Build history of the part. All positions in model axes, mm. A direction names the side the tool comes from. Round coordinates to 2 decimals unless told otherwise and drop trailing zeros. Loops run counter-clockwise (first coordinate to the right, second up) from the corner with the lowest first, then second, coordinate; pieces in that order, holes last. Notation, with made-up numbers: (52.5, -30) - (102.5, -30) arc R27 ccw to (102.5, -5) - close; hole circle Ø8 at (3, -28). An arc over 180 degrees is marked (long way). Put each result on its own line as item: value. Start each with the question number.
from build123d import *

# Parameters (mm, degrees)
PAD_DEPTH = 15
FILLET_R  = 1


with BuildPart() as part:
    # Sketch (on XZ_Plane of Origin) → Pad (new body)
    with BuildSketch(Plane.XZ):
        with BuildLine():
            Line((50, 0), (49.999618, 70.000262))
            Line((49.999618, 70.000262), (6.693182, 10.410738))
            Line((6.693182, 10.410738), (3.65564, 17.3888))
            Line((3.65564, 17.3888), (0, 17.3888))
            Line((0, 17.3888), (0, 1.424316))
            ThreePointArc((0, 1.424316), (0.417173, 0.417173), (1.424316, 0))
            Line((1.424316, 0), (7.946815, 0))
            Line((7.946815, 0), (40.015537, 44.126464))
            ThreePointArc((45.879073, 42.220854), (43.63951, 45.303564), (40.015537, 44.126464))
            Line((45.879073, 42.220854), (45.879073, 0))
            Line((45.879073, 0), (50, 0))
        make_face()
    extrude(amount=PAD_DEPTH)

    # Fillet
    fillet_edges = [part.edges().sort_by_distance(p)[0] for p in [
        (49.999618, -7.5, 70.000262),
    ]]
    fillet(fillet_edges, radius=FILLET_R)


solid = part.part
Item 1: Slice it at D-D (z = 5). Give the cut face in (x, y), plus the area to 3 significant figures.
Item 2: Two-plate mould, pull along X, no slides. Class faces 4 (the flat face through (27, -15, 27)), 5 (the cylindrical face through (0.406, -7.395, 0.428)), 6 (the flat face through (5.196, -7.395, 13.851)), 7 (the cylindrical face through (49.325, -7.605, 67.869)): pulls with the +X half, pulls with the -X half, needs draft (parallel to the pull), parting line crosses it, or undercut.
Item 3: Slice it at A-A (z = 14.5). Give the cut face in (x, y).
Item 4: Slice it at B-B (z = 24.5). Give the cut face in (x, y), plus the area to 3 significant figures.
Item 5: Drop flat-ended pins along their axis: pin 1 Ø8 at (y, z) = (-11, 53.5) entering from -X; pin 2 Ø2 at (x, y) = (29, -9.5) entering from -Z; pin 3 Ø5 at (x, y) = (31, -12.5) entering from -Z. Give the stop position or say it passes through.
Item 6: Drill centre lines: probe 1 along X at (y, z) = (-12.75, 16.5); probe 2 along X at (y, z) = (-5.75, 13.5); probe 3 along X at (y, z) = (-12.5, 20.5). Where is each one in solid material? Low to high. Write a range as [from, to].
Item 7: Which spindle directions (+Z, -Z, +X, -X, +Y, -Y) get a long thin tool onto all of the face, cutting with end or side? Do faces 1 (the flat face through (45.879, -7, 21)), 2 (the flat face through (2, -7, 17.389)), 3 (the flat face through (48, -7, 0)). Say none if no direction does.
Item 8: Slice it at C-C (y = -8.5). Give the cut face in (x, z), plus the area to 3 significant figures.
Computed values:
1. outline: (0, -15) - (11.58, -15) - (11.58, 0) - (0, 0) - close; (45.88, -15) - (50, -15) - (50, 0) - (45.88, 0) - close
1. area: 236 mm^2
2. face 4: needs draft
2. face 5: pulls with the -X half
2. face 6: undercut
2. face 7: parting line crosses it
3. outline: (0, -15) - (4.91, -15) - (4.91, 0) - (0, 0) - close; (9.67, -15) - (18.48, -15) - (18.48, 0) - (9.67, 0) - close; (45.88, -15) - (50, -15) - (50, 0) - (45.88, 0) - close
4. outline: (16.93, -15) - (25.75, -15) - (25.75, 0) - (16.93, 0) - close; (45.88, -15) - (50, -15) - (50, 0) - (45.88, 0) - close
4. area: 194 mm^2
5. pin 1: stops at x = 35.1
5. pin 2: stops at z = 27.59
5. pin 3: stops at z = 28.28
6. probe 1: x = [0, 4.04], [11.12, 19.94], [45.88, 50]
6. probe 2: x = [0, 5.35], [8.94, 17.76], [45.88, 50]
6. probe 3: x = [14.03, 22.85], [45.88, 50]
7. face 1: -Z, +Y, -Y
7. face 2: +Z, -X, +Y, -Y
7. face 3: -Z, +X, -X, +Y, -Y
8. outline: (0, 1.42) arc R1.42 ccw to (1.42, 0) - (7.95, 0) - (40.02, 44.13) arc R3.24 cw to (45.88, 42.22) - (45.88, 0) - (50, 0) - (50, 66.92) arc R1 ccw to (48.19, 67.51) - (6.69, 10.41) - (3.66, 17.39) - (0, 17.39) - close
8. area: 874 mm^2
